Model file for the job. Use its own axes, mm. Give positions to 0.01 mm unless a question says otherwise; leave off trailing zeros. Loops run counter-clockwise (first coordinate to the right, second up) from the corner with the lowest first, then second, coordinate; pieces in that order, holes last. Notation, with made-up numbers: M 70.5,46 L 128.5,46 A20 cw 128.5,54 Z; hole C -25.75,-6 d2. An arc over 180 degrees is marked long. Answer in a Markdown table with one row per item.
```python
from build123d import *

# Parameters (mm, degrees)
F1_DEPTH = 9


with BuildPart() as f1:
    # F0 (on Front) → F1 (new body)
    with BuildSketch(Plane.XZ):
        Polygon((0, 390), (0, 0), (720, 0), (720, 320), align=None)
        Polygon((-87.421968, 398.499358), (0, 0), (0, 390), align=None)
        Polygon((720, 320), (720, 0), (917.838265, 300.765724), align=None)
    extrude(amount=F1_DEPTH)


solid = f1.part
```
Q1. Drop flat-ended pins along their axis: pin 1 (5 mm diameter, centred on x = 291.5, z = 240.5, fed in from +Y); pin 2 (2 mm diameter, centred on x = 686.5, y = -5, fed in from +Z); pin 3 (4 mm diameter, centred on y = -8, z = 270.5, fed in from +X); pin 4 (1 mm diameter, centred on x = 59.5, y = -2.5, fed in from +Z). Give the stop position or say it passes through.
Reported:
| item | result |
|---|---|
| pin 1 | y = 0 |
| pin 2 | z = 323.35 |
| pin 3 | x = 899.25 |
| pin 4 | z = 384.26 |
Q2. Saw through at A-A (y = -5). Give the cut face in (x, z), and give its area (3 significant figures).
Reported:
| item | result |
|---|---|
| outline | M -87.42,398.5 L 0,0 L 720,0 L 917.84,300.77 Z |
| area | 304,000 mm² |
Q3. Saw through at B-B (x = 324). Give the cut face in (y, z), and give its area (3 significant figures).
Reported:
| item | result |
|---|---|
| outline | M -9,0 L 0,0 L 0,358.5 L -9,358.5 Z |
| area | 3,230 mm² |
Q4. Probe probe 1 along Z at (x, y) = (39, -7.25); probe 2 along X at (y, z) = (-1.75, 198); probe 3 along Z at (x, y) = (367, -0.75). List the from-to ranges inside material, lowest first.
Reported:
| item | result |
|---|---|
| probe 1 | 0 to 386.21 |
| probe 2 | -43.44 to 850.24 |
| probe 3 | 0 to 354.32 |
Q5. Saw through at C-C (z = 193). Give the cut face in (x, y), and give its area (3 significant figures).
Reported:
| item | result |
|---|---|
| outline | M -42.34,-9 L 846.95,-9 L 846.95,0 L -42.34,0 Z |
| area | 8,000 mm² |
